Build history of the part. All positions in model axes, mm. Face numbers are marked on the shaded views. A direction names the side the tool comes from. Round coordinates to 2 decimals unless told otherwise and drop trailing zeros. Write each loop counter-clockwise with the first axis right and the second up, starting at its lowest first coordinate (ties: lowest second). Pieces come first, ordered by that corner, then holes. Notation, with made-up numbers: (-16, 19) -> (-7, 19) arc R27 ccw to (-7, 43) -> close; hole circle Ø7 at (13, 41). An arc over 180 degrees is marked (long way). One line per question, with ' | ' between items.
from build123d import *

# Parameters (mm, degrees)
SKETCH_1_R               = 12
EXTRUDE_1_DEPTH          = 12
OTHER_1_2_OUTLINE_R      = 12
OTHER_1_2_OUTLINE_R_2    = 5
OTHER_1_2_DEPTH          = 12
OTHER_1_3_OUTLINE_R      = 5
OTHER_1_3_OUTLINE_R_2    = 4
OTHER_1_3_DEPTH          = 4
OTHER_START              = 8
OTHER_1_4_OUTLINE_R      = 5
OTHER_1_4_OUTLINE_R_2    = 4
OTHER_1_4_DEPTH          = 4
SKETCH_2_R               = 12
EXTRUDE_2_DEPTH          = 1
SKETCH_3_W               = 2
SKETCH_3_H               = 13
SKETCH_4_R               = 1
EXTRUDE_3_DEPTH          = 4
SKETCH_5_W               = 34.262916627
SKETCH_5_H               = 20.154656839
CUT_EXTRUDE_3_DEPTH      = 24.151673806
SKETCH_6_R               = 1.35
CUT_EXTRUDE_4_DEPTH      = 2
CUT_EXTRUDE_5_DEPTH      = 10
CUT_EXTRUDE_5_DEPTH_BACK = 10
SKETCH_7_R               = 4.05


with BuildPart() as part:
    # Sketch 1 → Extrude 1 (new body)
    with BuildSketch(Plane.XY):
        Circle(SKETCH_1_R)
    extrude(amount=EXTRUDE_1_DEPTH)

    # Other 1 2 outline → Other 1 2 (cut)
    with BuildSketch(Plane.XY):
        Circle(OTHER_1_2_OUTLINE_R)
        Circle(OTHER_1_2_OUTLINE_R_2, mode=Mode.SUBTRACT)
    extrude(amount=OTHER_1_2_DEPTH, mode=Mode.SUBTRACT)

    # Other 1 3 outline → Other 1 3 (cut)
    with BuildSketch(Plane.XY):
        Circle(OTHER_1_3_OUTLINE_R)
        Circle(OTHER_1_3_OUTLINE_R_2, mode=Mode.SUBTRACT)
    extrude(amount=OTHER_1_3_DEPTH, mode=Mode.SUBTRACT)

    # Other 1 4 outline → Other 1 4 (cut)
    with BuildSketch(Plane.XY.offset(OTHER_START)):
        Circle(OTHER_1_4_OUTLINE_R)
        Circle(OTHER_1_4_OUTLINE_R_2, mode=Mode.SUBTRACT)
    extrude(amount=OTHER_1_4_DEPTH, mode=Mode.SUBTRACT)


with BuildPart() as body_2:
    # Other 1: read off the stored shape, not the designer's step
    # Other 1 outline → Other 1 (revolve)
    with BuildSketch(Plane.XZ):
        with BuildLine():
            Line((12, 1), (12, 11))
            ThreePointArc((12, 11), (7, 6), (12, 1))
        make_face()
    revolve(axis=Axis((0, 0, 0), (0, 0, 1)))



with BuildPart() as body_2_2:
    # Sketch 2 → Extrude 2 (new body)
    with BuildSketch(Plane.XY):
        with Locations(Location((0, 0, 0), (0, 0, 270))):
            Circle(SKETCH_2_R)
    extrude(amount=-EXTRUDE_2_DEPTH)


with BuildPart() as body_2_1:
    add(body_2.part)

    add(body_2_2.part)  # Revolve 1 merges body 2 2
    # Sketch 3 → Revolve 1 (revolve)
    with BuildSketch(Plane(origin=(0, 0, 0), x_dir=(1, 0, 0), z_dir=(0, 1, 0))):
        with Locations((-13, -5.5)):
            Rectangle(SKETCH_3_W, SKETCH_3_H)
    revolve(axis=Axis((0, 0, 0), (0, 0, 1)))

    # Sketch 4 → Extrude 3 (add)
    with BuildSketch(Plane.XY):
        Circle(SKETCH_4_R)
    extrude(amount=EXTRUDE_3_DEPTH)

    # Sketch 5 → Cut-Extrude 3 (cut, through all)
    with BuildSketch(Plane(origin=(0, 0, 0), x_dir=(1, 0, 0), z_dir=(0, 1, 0))):
        with Locations((0.6382308, -6.140467699)):
            Rectangle(SKETCH_5_W, SKETCH_5_H)
    extrude(amount=-CUT_EXTRUDE_3_DEPTH, mode=Mode.SUBTRACT)

    # Sketch 6 → Cut-Extrude 4 (cut)
    with BuildSketch(Plane.XZ):
        with Locations(Location((10, 6, 0), (0, 0, 270))):
            Circle(SKETCH_6_R)
        with Locations(Location((-10, 6, 0), (0, 0, 270))):
            Circle(SKETCH_6_R)
    extrude(amount=-CUT_EXTRUDE_4_DEPTH, mode=Mode.SUBTRACT)

    # Sketch 7 → Cut-Extrude 5 (cut, two sides: drawn at the far end of the back side and taken through both)
    with BuildSketch(Plane.XY.offset(-CUT_EXTRUDE_5_DEPTH_BACK)):
        Circle(SKETCH_7_R)
    extrude(amount=CUT_EXTRUDE_5_DEPTH + CUT_EXTRUDE_5_DEPTH_BACK, mode=Mode.SUBTRACT)


solid = body_2_1.part
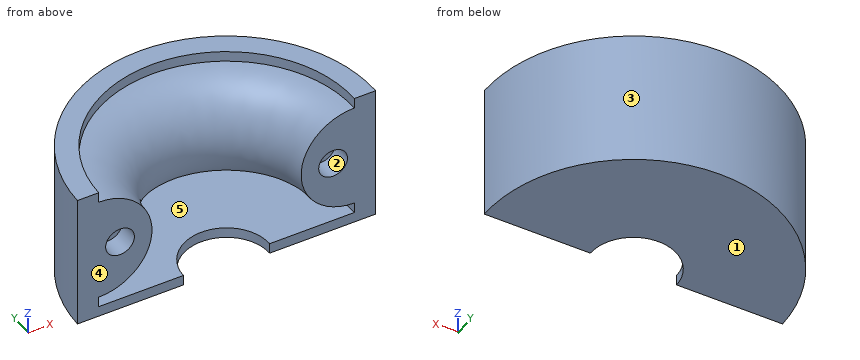
(1) Wall check: line 1 (X direction, y = 1.05, z = 6); line 2 (X direction, y = 1.2, z = 6); line 3 (Z direction, x = 5.25, y = 4.5). Give the ranges that are in metal, low to high. Write a range as from..to.
Calculated:
line 1: -13.96..-11.35, -8.65..-6.92, 6.92..8.65, 11.35..13.96 | line 2: -13.95..-11.35, -8.65..-6.9, 6.9..8.65, 11.35..13.95 | line 3: -1..0
(2) Slice it at B-B (y = 12.5). Write the cut outline in (x, z).
Calculated:
outline: (-6.3, -1) -> (6.3, -1) -> (6.3, 12) -> (-6.3, 12) -> close
(3) Slice it at C-C (z = 10). Write the cut outline in (x, y).
Calculated:
outline: (-14, 0) -> (-9, 0) arc R9 cw to (9, 0) -> (14, 0) arc R14 ccw to start
(4) Drop flat-ended pins along their axis: pin 1 (4.5 mm diameter, centred on x = -10, z = 6, fed in from +Y); pin 2 (1.6 mm diameter, centred on x = 10, z = 6, fed in from -Y); pin 3 (1 mm diameter, centred on y = 3, z = 8.5, fed in from -X) (3 decimals). Give the stop position or say it passes through.
Calculated:
pin 1: y = 11.66 | pin 2: y = 2 | pin 3: x = -13.775
(5) 3-axis set-ups, long thin cutter, end or side, ignore diameter. For the marked faces 1 and 2: which of +Z, -Z, +X, -X, +Y, -Y reach the whole face in a straight line?
Calculated:
face 1: -Z, +X, -X, +Y, -Y | face 2: -Y
(6) Slice it at A-A (z = 6). Write the cut outline in (x, y).
Calculated:
outline: (-14, 0) -> (-11.35, 0) -> (-11.35, 2) -> (-8.65, 2) -> (-8.65, 0) -> (-7, 0) arc R7 cw to (7, 0) -> (8.65, 0) -> (8.65, 2) -> (11.35, 2) -> (11.35, 0) -> (14, 0) arc R14 ccw to start
(7) Mould opens along X. For the marked faces 3, 4 and 5 say: pulls with the +X half, pulls with the -X half, needs draft (parallel to the pull), parting line crosses it, or undercut.
Calculated:
face 3: parting line crosses it | face 4: needs draft | face 5: undercut
